Work out the finished part from the listing and answer in its coordinate system (mm). A direction names the side the tool comes from. Give positions to 0.01 mm unless a question says otherwise; leave off trailing zeros. Loops run counter-clockwise (first coordinate to the right, second up) from the corner with the lowest first, then second, coordinate; pieces in that order, holes last. Notation, with made-up numbers: M -10.5,25 L 9.5,25 A15 ccw 9.5,53 Z; hole C 54,-28 d10. An arc over 180 degrees is marked long. Use a Markdown table: item, result.
```python
from build123d import *

# Parameters (mm, degrees)
ESQUISSE1_W             = 11.5
ESQUISSE1_H             = 32.5
BOSS_EXTRU_1_DEPTH      = 18.5
ESQUISSE4_W             = 9.5
ESQUISSE4_H             = 32
ENL_V_MAT_EXTRU_1_DEPTH = 16.5
ESQUISSE5_W             = 9.5
ESQUISSE5_H             = 5
BOSS_EXTRU_2_DEPTH      = 16
ESQUISSE6_R             = 0.9
ENL_V_MAT_EXTRU_2_DEPTH = 6
ESQUISSE7_W             = 11.5
ESQUISSE7_H             = 2
BOSS_EXTRU_3_DEPTH      = 21
ESQUISSE9_W             = 9.5
ESQUISSE9_H             = 5
BOSS_EXTRU_4_DEPTH      = 16
ESQUISSE10_R            = 0.9
ENL_V_MAT_EXTRU_3_DEPTH = 7
ESQUISSE11_W            = 9.5
ESQUISSE11_H            = 7
ENL_V_MAT_EXTRU_4_DEPTH = 7
ESQUISSE12_W            = 11.5
ESQUISSE12_H            = 3
BOSS_EXTRU_5_DEPTH      = 30
ESQUISSE13_R            = 2.5
ENL_V_MAT_EXTRU_5_DEPTH = 10
ESQUISSE15_W            = 8.5
ESQUISSE15_H            = 3
ENL_V_MAT_EXTRU_6_DEPTH = 10


with BuildPart() as part:
    # Esquisse1 → Boss.-Extru.1 (new body)
    with BuildSketch(Plane.XY):
        with Locations((-5.75, 16.25)):
            Rectangle(ESQUISSE1_W, ESQUISSE1_H)
    extrude(amount=BOSS_EXTRU_1_DEPTH)

    # Esquisse4 → Enlèv. mat.-Extru.1 (cut)
    with BuildSketch(Plane.XY.offset(18.5)):
        with Locations((-5.75, 16)):
            Rectangle(ESQUISSE4_W, ESQUISSE4_H)
    extrude(amount=-ENL_V_MAT_EXTRU_1_DEPTH, mode=Mode.SUBTRACT)

    # Esquisse5 → Boss.-Extru.2 (add)
    with BuildSketch(Plane.XY.offset(2)):
        with Locations((-5.75, 29.5)):
            Rectangle(ESQUISSE5_W, ESQUISSE5_H)
    extrude(amount=BOSS_EXTRU_2_DEPTH)

    # Esquisse6 → Enlèv. mat.-Extru.2 (cut)
    with BuildSketch(Plane.XY.offset(18)):
        with Locations((-5.75, 30)):
            Circle(ESQUISSE6_R)
    extrude(amount=-ENL_V_MAT_EXTRU_2_DEPTH, mode=Mode.SUBTRACT)

    # Esquisse7 → Boss.-Extru.3 (add)
    with BuildSketch(Plane.XZ):
        with Locations((-5.75, 1)):
            Rectangle(ESQUISSE7_W, ESQUISSE7_H)
    extrude(amount=BOSS_EXTRU_3_DEPTH)

    # Esquisse9 → Boss.-Extru.4 (add)
    with BuildSketch(Plane.XY.offset(2)):
        with Locations((-5.75, 2.5)):
            Rectangle(ESQUISSE9_W, ESQUISSE9_H)
    extrude(amount=BOSS_EXTRU_4_DEPTH)

    # Esquisse10 → Enlèv. mat.-Extru.3 (cut)
    with BuildSketch(Plane.XY.offset(18)):
        with Locations((-5.75, 2)):
            Circle(ESQUISSE10_R)
    extrude(amount=-ENL_V_MAT_EXTRU_3_DEPTH, mode=Mode.SUBTRACT)

    # Esquisse11 → Enlèv. mat.-Extru.4 (cut)
    with BuildSketch(Plane.XZ):
        with Locations((-5.75, 5.5)):
            Rectangle(ESQUISSE11_W, ESQUISSE11_H)
    extrude(amount=-ENL_V_MAT_EXTRU_4_DEPTH, mode=Mode.SUBTRACT)

    # Esquisse12 → Boss.-Extru.5 (add)
    with BuildSketch(Plane.XY.offset(2)):
        with Locations((-5.75, -19.5)):
            Rectangle(ESQUISSE12_W, ESQUISSE12_H)
    extrude(amount=BOSS_EXTRU_5_DEPTH)

    # Esquisse13 → Enlèv. mat.-Extru.5 (cut)
    with BuildSketch(Plane.XZ.offset(21)):
        with Locations((-5.75, 12)):
            Circle(ESQUISSE13_R)
        with Locations((-5.75, 25)):
            Circle(ESQUISSE13_R)
    extrude(amount=-ENL_V_MAT_EXTRU_5_DEPTH, mode=Mode.SUBTRACT)

    # Esquisse15 → Enlèv. mat.-Extru.6 (cut)
    with BuildSketch(Plane.XZ.offset(21)):
        with Locations((-5.75, 4.5)):
            Rectangle(ESQUISSE15_W, ESQUISSE15_H)
    extrude(amount=-ENL_V_MAT_EXTRU_6_DEPTH, mode=Mode.SUBTRACT)


solid = part.part
```
(1) A cutting plane is placed at B-B (y = 2). Write down the section's boundary in (x, z).
Entries:
| item | result |
|---|---|
| outline | M -11.5,0 L 0,0 L 0,18.5 L -1,18.5 L -1,18 L -4.85,18 L -4.85,11 L -6.65,11 L -6.65,18 L -10.5,18 L -10.5,18.5 L -11.5,18.5 Z; hole M -10.5,2 L -1,2 L -1,9 L -10.5,9 Z |
(2) A cutting plane is placed at C-C (z = 25). Write down the section's boundary in (x, y).
Entries:
| item | result |
|---|---|
| outline | M -11.5,-21 L -8.25,-21 L -8.25,-18 L -11.5,-18 Z; M -3.25,-21 L 0,-21 L 0,-18 L -3.25,-18 Z |
(3) Consider probe 1 along Z at (x, y) = (-5.75, -20.3); probe 2 along Y at (x, z) = (-7.5, 9.5); probe 3 along Y at (x, z) = (-5.75, 12.75). Determine where each line is inside the solid, lowest interval first. Write a range as [from, to].
Entries:
| item | result |
|---|---|
| probe 1 | z = [0, 3], [6, 9.5], [14.5, 22.5], [27.5, 32] |
| probe 2 | y = [-21, -18], [0, 5], [27, 32.5] |
| probe 3 | y = [0, 1.1], [2.9, 5], [27, 29.1], [30.9, 32.5] |
(4) A cutting plane is placed at D-D (y = 24.5). Write down the section's boundary in (x, z).
Entries:
| item | result |
|---|---|
| outline | M -11.5,0 L 0,0 L 0,18.5 L -1,18.5 L -1,2 L -10.5,2 L -10.5,18.5 L -11.5,18.5 Z |
(5) Which of the six approach directions +Z, -Z, +X, -X, +Y, -Y give full straight-line access (tool end or side, diameter ignored) to faces 4 (the flat face through (-6, 2, 9)), 5 (the cylindrical face through (-4.6, -19.52, 9.78)), 6 (the flat face through (-6, 32.5, 9)), 7 (the flat face through (-11.5, 5, 9)), 8 (the cylindrical face through (-6.65, 2.04, 14.55))?
Entries:
| item | result |
|---|---|
| face 4 | none |
| face 5 | -Y |
| face 6 | +Z, -Z, +X, -X, +Y |
| face 7 | +Z, -Z, -X, +Y, -Y |
| face 8 | +Z |
(6) The mould has two halves that part along Y. Classify faces 1 (the flat face through (-6, -21, 16)), 2 (the flat face through (-1.5, -20, 4)), 3 (the flat face through (-6, 2, 11)): released by +Y, released by -Y, zero draft, split by the parting line, or undercut.
Entries:
| item | result |
|---|---|
| face 1 | released by -Y |
| face 2 | zero draft |
| face 3 | undercut |
(7) Given P1, Ø2.5, axis at x = -4, y = 3.5, coming from the +Z side; P2, Ø5, axis at x = -7, y = 13.5, coming from the +Z side; P3, Ø0.5, axis at x = -5.5, y = 2.5, coming from the +Z side, each flat-ended and moving along its own axis, determine where each tip first touches the part or whether it passes through.
Entries:
| item | result |
|---|---|
| P1 | stops at z = 18 |
| P2 | stops at z = 2 |
| P3 | stops at z = 11 |
(8) A cutting plane is placed at A-A (x = -5.75). Count the separate pieces of the cut face and the enclosed holes in it, and give its area (3 significant figures).
Entries:
| item | result |
|---|---|
| separate pieces | 5 |
| enclosed holes | 0 |
| area | 268 mm² |
